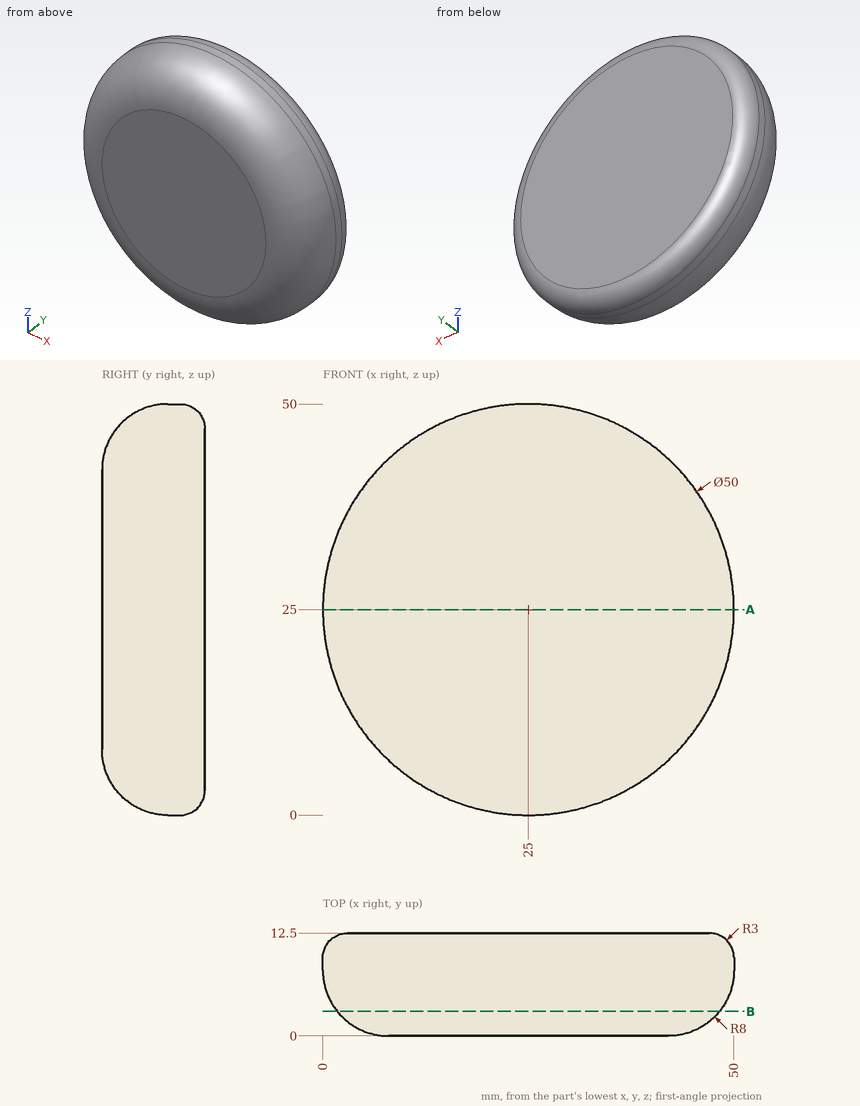
Here's the drawing with two shaded views (mm, measured from the low corner). I have some questions. Coordinates: 2 decimals unless noted, no trailing zeros. Loops run counter-clockwise (first coordinate to the right, second up) from the corner with the lowest first, then second, coordinate; pieces in that order, holes last. Notation, with made-up numbers: M -13,-8 L 39,-8 A18 ccw 39,23 Z; hole C 5,-30 d8. An arc over 180 degrees is marked long. Answer as CSV lines item,"result". Start each with the question number.
1. For pin 1 Ø4 at (y, z) = (11, 17) entering from +X; pin 2 Ø1.5 at (y, z) = (5, 33) entering from +X; pin 3 Ø1.5 at (x, y) = (45, 7) entering from +Z, each with a flat end and sliding along its axis, tell me the tip position at first contact or that it passes through.
2. Suppose I cut it at A-A, the plane z = 25. List the corners of the cut face in (x, y) for me.
3. If I drill on probe 1 along Y at (x, z) = (32.5, 9.5); probe 2 along X at (y, z) = (1, 20); probe 3 along Z at (x, y) = (3, 4.75), over which ranges is the centre line in solid material (lowest first)? Write a range as [from, to].
4. Suppose I cut it at B-B, the plane y = 3. List the corners of the cut face in (x, z) for me (3 decimals), plus the area to 3 significant figures.
Output:
1,pin 1,"stops at x = 49.16"
1,pin 2,"stops at x = 48.45"
1,pin 3,"stops at z = 40.86"
2,outline,"M 0,8 A8 ccw 8,0 L 42,0 A8 ccw 50,8 L 50,9.5 A3 ccw 47,12.5 L 3,12.5 A3 ccw 0,9.5 Z"
3,probe 1,"y = [0, 12.5]"
3,probe 2,"x = [4.73, 45.27]"
3,probe 3,"z = [14.66, 35.34]"
4,outline,"C 25,25 d46.49"
4,area,"1,700 mm^2"
